Here's how the part is built. I have some questions about the finished solid (model axes, mm). A direction names the side the tool comes from. Coordinates: 2 decimals unless noted, no trailing zeros. Loops run counter-clockwise (first coordinate to the right, second up) from the corner with the lowest first, then second, coordinate; pieces in that order, holes last.
```python
from build123d import *

# Parameters (mm, degrees)
F0_W     = 1348.74
F0_H     = 685.8
F1_DEPTH = 25.4
F3_W     = 50.8
F3_H     = 317.5
F4_DEPTH = 38.1
F5_W     = 50.8
F5_H     = 76.2
F6_DEPTH = 660.4


with BuildPart() as f1:
    # F0 (on Top) → F1 (new body)
    with BuildSketch(Plane.XY):
        Rectangle(F0_W, F0_H)
    extrude(amount=F1_DEPTH)

    # F3 (on face) → F4 (join)
    with BuildSketch(Plane.XY.offset(25.4)):
        with Locations((-623.57, 44.45)):
            Rectangle(F3_W, F3_H)
        with Locations((623.57, 44.45)):
            Rectangle(F3_W, F3_H)
    extrude(amount=F4_DEPTH)

    # F5 (on face) → F6 (join)
    with BuildSketch(Plane.XY.offset(25.4)):
        with Locations((-623.57, -152.4)):
            Rectangle(F5_W, F5_H)
        with Locations((623.57, -152.4)):
            Rectangle(F5_W, F5_H)
    extrude(amount=F6_DEPTH)


solid = f1.part
```
1. I want a section at A-A (z = 218). Please give me the cut outline in (x, y).
2. For pin 1 (1.5 mm diameter, centred on x = 191.5, y = 273, fed in from +Z); pin 2 (5 mm diameter, centred on y = -112, z = 484.5, fed in from +X); pin 3 (15 mm diameter, centred on x = 631, z = 489.5, fed in from +Y), each with a flat end and sliding along its axis, tell me the tip position at first contact or that it passes through.
3. I need wall thicknesses on line 1 along X through (y, z) = (-127.5, 493); line 2 along Z through (x, y) = (339, 313.5). Which ranges of each line are inside material? Lowest first, please.
4. We'd pull the mould along X, two halves only. Please class faces 1 (the flat face through (-624, 47, 63.5)), 2 (the flat face through (-598.17, -126, 281)), 3 (the flat face through (-648.97, -126, 281)): +X half, -X half, draft (parallel to the pull), parting line (faces both ways), or undercut.
5. I want a section at B-B (y = 26.5). Please give me the cut outline in (x, z).
6. On a 3-axis mill with a long thin cutter (end or side, diameter ignored), from which of +Z, -Z, +X, -X, +Y, -Y can I reach the whole of each face in a straight line? I mean faces 4 (the flat face through (623, -190.5, 351)), 5 (the flat face through (623, -152, 685.8)), 6 (the flat face through (598.17, -126, 281)), 7 (the flat face through (648.97, -126, 281)), 8 (the flat face through (-624, 203.2, 44)). Say none if no direction works.
7. I want a section at C-C (x = 168.5). Please give me the cut outline in (y, z).
Response values:
1. outline: (-648.97, -190.5) - (-598.17, -190.5) - (-598.17, -114.3) - (-648.97, -114.3) - close; (598.17, -190.5) - (648.97, -190.5) - (648.97, -114.3) - (598.17, -114.3) - close
2. pin 1: stops at z = 25.4
2. pin 2: stops at x = 648.97
2. pin 3: stops at y = -114.3
3. line 1: x = -648.97 to -598.17, 598.17 to 648.97
3. line 2: z = 0 to 25.4
4. face 1: draft
4. face 2: undercut
4. face 3: -X half
5. outline: (-674.37, 0) - (674.37, 0) - (674.37, 25.4) - (648.97, 25.4) - (648.97, 63.5) - (598.17, 63.5) - (598.17, 25.4) - (-598.17, 25.4) - (-598.17, 63.5) - (-648.97, 63.5) - (-648.97, 25.4) - (-674.37, 25.4) - close
6. face 4: +Z, +X, -X, -Y
6. face 5: +Z, +X, -X, +Y, -Y
6. face 6: +Z, +Y, -Y
6. face 7: +Z, +X, +Y, -Y
6. face 8: +Z, +X, -X, +Y
7. outline: (-342.9, 0) - (342.9, 0) - (342.9, 25.4) - (-342.9, 25.4) - close
